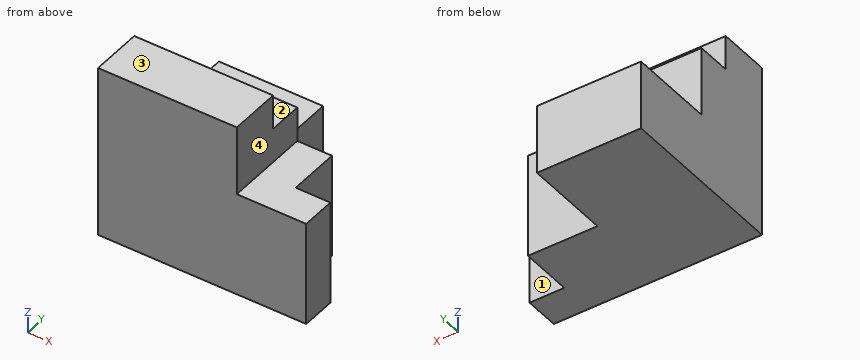
```python
from build123d import *

# Parameters (mm, degrees)
BOSS_EXTRUDE1_DEPTH = 31.75
SKETCH3_W           = 12.7
SKETCH3_H           = 38.1
CUT_EXTRUDE3_DEPTH  = 19.05
SKETCH6_W           = 50.8
SKETCH6_H           = 12.7
CUT_EXTRUDE5_DEPTH  = 44.45
SKETCH7_W           = 50.8
SKETCH7_H           = 19.05
BOSS_EXTRUDE2_DEPTH = 12.7
SKETCH8_W           = 38.1
SKETCH8_H           = 25.4
BOSS_EXTRUDE3_DEPTH = 31.75


with BuildPart() as part:
    # Sketch1 → Boss-Extrude1 (new body)
    with BuildSketch(Plane(origin=(0, 0, 0), x_dir=(1, 0, 0), z_dir=(0, 1, 0))):
        Polygon((0, 0), (50.8, 0), (50.8, 25.4), (76.2, 25.4), (76.2, 63.5), (0, 63.5), align=None)
    extrude(amount=BOSS_EXTRUDE1_DEPTH)

    # Sketch3 → Cut-Extrude3 (cut)
    with BuildSketch(Plane(origin=(0, 31.75, 0), x_dir=(1, 0, 0), z_dir=(0, 1, 0))):
        with Locations((69.85, 44.45)):
            Rectangle(SKETCH3_W, SKETCH3_H)
    extrude(amount=-CUT_EXTRUDE3_DEPTH, mode=Mode.SUBTRACT)

    # Sketch6 → Cut-Extrude5 (cut)
    with BuildSketch(Plane.XZ):
        with Locations((25.4, -6.35)):
            Rectangle(SKETCH6_W, SKETCH6_H)
    extrude(amount=-CUT_EXTRUDE5_DEPTH, mode=Mode.SUBTRACT)

    # Sketch7 → Boss-Extrude2 (add)
    with BuildSketch(Plane.XY.offset(-12.7)):
        with Locations((25.4, 9.525)):
            Rectangle(SKETCH7_W, SKETCH7_H)
    extrude(amount=BOSS_EXTRUDE2_DEPTH)

    # Sketch8 → Boss-Extrude3 (add)
    with BuildSketch(Plane(origin=(0, 31.75, 0), x_dir=(1, 0, 0), z_dir=(0, 1, 0))):
        with Locations((19.05, 50.8)):
            Rectangle(SKETCH8_W, SKETCH8_H)
    extrude(amount=BOSS_EXTRUDE3_DEPTH)


solid = part.part
```
Check sheet for the modelled part. Datum: model origin and axes. Units: mm. Face numbers are marked on the shaded views. A direction names the side the tool comes from. Round coordinates to 2 decimals unless told otherwise and drop trailing zeros. Write each loop counter-clockwise with the first axis right and the second up, starting at its lowest first coordinate (ties: lowest second). Pieces come first, ordered by that corner, then holes. Notation, with made-up numbers: M -29.75,39.25 L -4.75,39.25 A28 cw -4.75,57.25 Z; hole C 70,67.5 d5. An arc over 180 degrees is marked long. Write item = value, one per line. Start each with the question number.
1. Section check B-B, the plane y = 9. Record the cut outline in (x, z), then the cut area to 3 significant figures.
2. Scan lines: line 1 (X direction, y = 37.5, z = -50); line 2 (X direction, y = 23.5, z = -26); line 3 (Y direction, x = 10.5, z = -8). Record each from-to range of solid material in increasing order. Write a range as [from, to].
3. Section check C-C, the plane z = -43.5. Record the cut outline in (x, y).
4. Gauge pin test, flat ends, axial feed: pin 1 (12 mm diameter, centred on x = 45.5, y = 49, fed in from -Z); pin 2 (2 mm diameter, centred on x = 21.5, y = 43, fed in from +Z); pin 3 (10 mm diameter, centred on x = 29, z = -6.5, fed in from +Y); pin 4 (20.5 mm diameter, centred on y = 50.5, z = -55.5, fed in from +X). Record the tip position at first contact, or that the pin passes through.
5. Section check D-D, the plane x = 12. Record the cut outline in (y, z).
6. Tool access check on the marked faces 1, 2, 3 and 4. Record the directions out of +Z, -Z, +X, -X, +Y, -Y that give a thin tool (end or side, any length) a straight path to the whole face; none if there is none.
7. Section check A-A, the plane x = 45.5. Record the cut outline in (y, z).
Results found:
q1.outline = M 0,-63.5 L 76.2,-63.5 L 76.2,-25.4 L 50.8,-25.4 L 50.8,0 L 0,0 Z
q1.area = 4,190 mm^2
q2.line_1 = [0, 38.1]
q2.line_2 = [0, 63.5]
q2.line_3 = [0, 19.05]
q3.outline = M 0,0 L 76.2,0 L 76.2,12.7 L 63.5,12.7 L 63.5,31.75 L 38.1,31.75 L 38.1,63.5 L 0,63.5 Z
q4.pin_1 = through
q4.pin_2 = -38.1
q4.pin_3 = 19.05
q4.pin_4 = 38.1
q5.outline = M 0,-63.5 L 63.5,-63.5 L 63.5,-38.1 L 31.75,-38.1 L 31.75,-12.7 L 19.05,-12.7 L 19.05,0 L 0,0 Z
q6.face_1 = +Z, -Z, +X, +Y
q6.face_2 = +Z, +X, -X, +Y
q6.face_3 = +Z, +X, -X, +Y, -Y
q6.face_4 = +Z, +X, +Y, -Y
q7.outline = M 0,-63.5 L 31.75,-63.5 L 31.75,-12.7 L 19.05,-12.7 L 19.05,0 L 0,0 Z
